Autodesk Inventor part; units mm, degrees
ref_plane "YZ Plane" through (0, 0, 0) normal (1, 0, 0) x (0, 1, 0)
ref_plane "XZ Plane" through (0, 0, 0) normal (0, 1, 0) x (-1, 0, 0)
ref_plane "XY Plane" through (0, 0, 0) normal (0, 0, 1) x (1, 0, 0)
sketch "Sketch2" plane through (0, 0, 0) normal (1, 0, 0) x (0, 1, 0)
  circle A0 centre (0, 0) radius 14.2875
  dimension "d0" = 28.575
extrude "Extrusion1" add sketch "Sketch2" along normal mid plane 76.2
sketch "Sketch3" plane through (38.1, 0, 0) normal (1, 0, 0) x (0, 0, -1)
  circle A0 centre (0, 0) radius 14.2875
  circle A1 centre (0, 0) radius 28.575
  dimension "d3" = 57.15
extrude "Extrusion2" add sketch "Sketch3" along normal blind 76.2 contours A0 | A1
mirror "Mirror1" about plane through (0, 0, 0) normal (1, 0, 0) of "Extrusion2"
properties part number "Roller"
The model under review builds one solid part; all positions refer to its coordinate system, in mm. A direction names the side the tool comes from. Round coordinates to 2 decimals unless told otherwise and drop trailing zeros. Order: outer loops, then holes, each group sorted by start corner. A loop starts at its lowest first (then second) coordinate and runs counter-clockwise, first axis right, second up. Notation, with made-up numbers: (11, 73.5) -> (29, 73.5) arc R17 cw to (29, 86.5) -> close; hole circle Ø7 at (-10.75, 64). An arc over 180 degrees is marked (long way). One line per item, written item: value. Start each with the question number.
Q1. Take a section at A-A (z = -22). Write out the cut boundary in (x, y), and give its area (3 significant figures).
Q2. Mouldability with a two-part tool opening along X and no side actions: class faces 1 (the face through (0.533, -14.274, 0.628)), 2 (the face through (-114.3, 0, 0)), 3 (the face through (-75.667, 1.256, 28.547)) as released by +X, released by -X, zero draft, split by the parting line, or undercut.
Q3. Machinability: for faces 4 (the face through (75.667, -1.256, 28.547)), 5 (the face through (38.1, 7, 13)), which of the approach directions +Z, -Z, +X, -X, +Y, -Y give a long, thin tool a straight path to every point of the face, cutting with its end or side? Answer none if there is none.
Q4. Take a section at D-D (x = -53). Write out the cut boundary in (y, z) (3 decimals), and give its area (3 significant figures).
Q5. Clearance check with flat-ended pins moving along their axes: pin 1 Ø2 at (x, y) = (68, 11) entering from -Z; pin 2 Ø1.5 at (x, z) = (25, -1.5) entering from +Y; pin 3 Ø3 at (x, y) = (7, -14) entering from +Z. State where each tip first meets the part, or that it passes through.
Q6. Take a section at B-B (y = 0). Write out the cut boundary in (x, z) (1 decimal).
Q7. Wall thickness on line 1 (X direction, y = 14.5, z = 11); line 2 (Z direction, x = -87, y = 0.5); line 3 (Z direction, x = -16, y = -1): over which ranges is each line inside the solid? List them lowest first.
Reported:
1. outline: (-114.3, -18.24) -> (-38.1, -18.24) -> (-38.1, 18.24) -> (-114.3, 18.24) -> close; (38.1, -18.24) -> (114.3, -18.24) -> (114.3, 18.24) -> (38.1, 18.24) -> close
1. area: 5,560 mm2
2. face 1: undercut
2. face 2: released by -X
2. face 3: zero draft
3. face 4: +X, -X
3. face 5: none
4. outline: circle Ø57.15 at (0, 0)
4. area: 2,570 mm2
5. pin 1: stops at z = -26.77
5. pin 2: stops at y = 14.27
5. pin 3: stops at z = 6.92
6. outline: (-114.3, -28.6) -> (-38.1, -28.6) -> (-38.1, -14.3) -> (38.1, -14.3) -> (38.1, -28.6) -> (114.3, -28.6) -> (114.3, 28.6) -> (38.1, 28.6) -> (38.1, 14.3) -> (-38.1, 14.3) -> (-38.1, 28.6) -> (-114.3, 28.6) -> close
7. line 1: x = -114.3 to -38.1, 38.1 to 114.3
7. line 2: z = -28.57 to 28.57
7. line 3: z = -14.25 to 14.25
